from build123d import *

# Parameters (mm, degrees)
SKETCH_1_W                 = 40
SKETCH_1_H                 = 22
EXTRUDE_1_DEPTH            = 6
M3_TAPPED_HOLE1_AT_2_COUNT = 2
M3_TAPPED_HOLE1_AT_2_PITCH = 33
CHAMFER_1_SIZE             = 0.5
SKETCH_5_R                 = 7.5
CUT_EXTRUDE_2_DEPTH        = 12
CHAMFER1_SIZE              = 0.5
SKETCH2_W                  = 25
SKETCH2_H                  = 22
EXTRUDE2_DEPTH             = 6.5
CHAMFER2_SIZE              = 1
CHAMFER3_SIZE              = 3


with BuildPart() as part:
    # 草图1 → 拉伸1 (new, symmetric)
    with BuildSketch(Plane.XY):
        Rectangle(SKETCH_1_W, SKETCH_1_H)
    extrude(amount=EXTRUDE_1_DEPTH, both=True)

    # 草图4 → M3 Tapped Hole1 (revolve, cut)
    with BuildSketch(Plane(origin=(-16.5, -11, 3.5), x_dir=(0, 0, -1), z_dir=(1, 0, 0))):
        Polygon((0, 0), (0, 10.251075774), (1.25, 9.5), (1.25, 0), align=None)
    m3_tapped_hole1 = revolve(axis=Axis((-16.5, -17.35, 3.5), (0, 1, 0)), mode=Mode.SUBTRACT)

    # M3 Tapped Hole1 at 2: M3 Tapped Hole1 ×2
    with Locations(*[(i * M3_TAPPED_HOLE1_AT_2_PITCH, 0, 0) for i in range(1, M3_TAPPED_HOLE1_AT_2_COUNT)]):
        add(m3_tapped_hole1, mode=Mode.SUBTRACT)

    # 倒角1
    chamfer_1_edges = [part.edges().sort_by_distance(p)[0] for p in [
        (16.5, -11, 4.75),
        (-16.5, -11, 4.75),
    ]]
    chamfer(chamfer_1_edges, length=CHAMFER_1_SIZE)

    # 草图5 → 拉伸2 (cut)
    with BuildSketch(Plane.XY.offset(6)):
        Circle(SKETCH_5_R)
    extrude(amount=-CUT_EXTRUDE_2_DEPTH, mode=Mode.SUBTRACT)

    # Mirror1: M3 Tapped Hole1 across plane
    add(m3_tapped_hole1.mirror(Plane.XY), mode=Mode.SUBTRACT)

    # Mirror1 copy 1 sketch → Mirror1 copy 1 (revolve, cut)
    with BuildSketch(Plane(origin=(16.5, -11, -3.5), x_dir=(0, 0, 1), z_dir=(1, 0, 0))):
        Polygon((0, 0), (0, -10.251075774), (1.25, -9.5), (1.25, 0), align=None)
    revolve(axis=Axis((16.5, -17.35, -3.5), (0, -1, 0)), mode=Mode.SUBTRACT)

    # Chamfer1
    chamfer1_edges = [part.edges().sort_by_distance(p)[0] for p in [
        (16.5, -11, -4.75),
        (-16.5, -11, -4.75),
    ]]
    chamfer(chamfer1_edges, length=CHAMFER1_SIZE)

    # Sketch2 → Extrude2 (cut)
    with BuildSketch(Plane(origin=(0, 0, -6), x_dir=(-1, 0, 0), z_dir=(0, 0, -1))):
        Rectangle(SKETCH2_W, SKETCH2_H)
    extrude(amount=-EXTRUDE2_DEPTH, mode=Mode.SUBTRACT)

    # Chamfer2
    chamfer2_edges = [part.edges().sort_by_distance(p)[0] for p in [
        (12.5, 0, -6),
        (-12.5, 0, -6),
    ]]
    chamfer(chamfer2_edges, length=CHAMFER2_SIZE)

    # Chamfer3
    chamfer3_edges = [part.edges().sort_by_distance(p)[0] for p in [
        (20, 0, 6),
        (-20, 0, 6),
        (20, 0, -6),
        (-20, 0, -6),
    ]]
    chamfer(chamfer3_edges, length=CHAMFER3_SIZE)


solid = part.part
Geometry check sheet. Reference: the model listing, model coordinates, mm. A direction names the side the tool comes from. Give positions to 0.01 mm unless a question says otherwise; leave off trailing zeros. Order: outer loops, then holes, each group sorted by start corner. A loop starts at its lowest first (then second) coordinate and runs counter-clockwise, first axis right, second up.
1) Cross-section at C-C (z = -0.25). Record the boundary of the cut face in (x, y), then the cut area to 3 significant figures.
Results are:
outline: (-20, -11) - (-12.5, -11) - (-12.5, 11) - (-20, 11) - close; (12.5, -11) - (20, -11) - (20, 11) - (12.5, 11) - close
area: 330 mm2
2) Cross-section at A-A (x = 0). Record the boundary of the cut face in (y, z), then the cut area to 3 significant figures.
Results are:
outline: (-11, 0.5) - (-7.5, 0.5) - (-7.5, 6) - (-11, 6) - close; (7.5, 0.5) - (11, 0.5) - (11, 6) - (7.5, 6) - close
area: 38.5 mm2
3) Draft check along X on faces 4 (the conical face through (16.69, -0.88, 3.4)), 5 (the flat face through (-19, 0, 4)), 6 (the flat face through (-8, 0, 6)). Enter one of: released by +X, released by -X, zero draft, split by the parting line, or undercut.
Results are:
face 4: undercut
face 5: released by -X
face 6: zero draft
4) Gauge pin test, flat ends, axial feed: pin 1 (5 mm diameter, centred on x = -7.5, z = 0, fed in from +Y); pin 2 (9 mm diameter, centred on x = 0, y = 0, fed in from -Z); pin 3 (3 mm diameter, centred on x = 16.5, z = 3.5, fed in from -Y); pin 4 (11 mm diameter, centred on x = -1, y = 4.5, fed in from -Z). Record the tip position at first contact, or that the pin passes through.
Results are:
pin 1: stops at y = 11
pin 2: passes through
pin 3: stops at y = -10.75
pin 4: stops at z = 0.5
5) Tool access check on faces 1 (the flat face through (-13, -0.2, -5.5)), 2 (the flat face through (0, -11, 1)), 3 (the cylindrical face through (-17.554, -6.063, 2.828)). Record the directions out of +Z, -Z, +X, -X, +Y, -Y that give a thin tool (end or side, any length) a straight path to the whole face; none if there is none.
Results are:
face 1: -Z, +Y, -Y
face 2: +Z, -Z, +X, -X, -Y
face 3: -Y
6) Material ranges on probe 1 along Z at (x, y) = (-16.5, -6.75); probe 2 along X at (y, z) = (-5, 3.5); probe 3 along X at (y, z) = (-4, -3.5), recorded low to high.
Results are:
probe 1: z = -6 to -4.75, -2.25 to 2.25, 4.75 to 6
probe 2: x = -19.5 to -17.75, -15.25 to -5.59, 5.59 to 15.25, 17.75 to 19.5
probe 3: x = -19.5 to -17.75, -15.25 to -12.5, 12.5 to 15.25, 17.75 to 19.5
7) Cross-section at B-B (y = 0). Record the boundary of the cut face in (x, z), then the cut area to 3 significant figures.
Results are:
outline: (-20, -3) - (-17, -6) - (-13.5, -6) - (-12.5, -5) - (-12.5, 0.5) - (-7.5, 0.5) - (-7.5, 6) - (-17, 6) - (-20, 3) - close; (7.5, 0.5) - (12.5, 0.5) - (12.5, -5) - (13.5, -6) - (17, -6) - (20, -3) - (20, 3) - (17, 6) - (7.5, 6) - close
area: 216 mm2
8) Cross-section at D-D (y = -2.75). Record the boundary of the cut face in (x, z), then the cut area to 3 significant figures.
Results are:
outline: (-20, -3) - (-17, -6) - (-13.5, -6) - (-12.5, -5) - (-12.5, 0.5) - (-6.98, 0.5) - (-6.98, 6) - (-17, 6) - (-20, 3) - close; (6.98, 0.5) - (12.5, 0.5) - (12.5, -5) - (13.5, -6) - (17, -6) - (20, -3) - (20, 3) - (17, 6) - (6.98, 6) - close; hole circle Ø2.5 at (-16.5, -3.5); hole circle Ø2.5 at (-16.5, 3.5); hole circle Ø2.5 at (16.5, -3.5); hole circle Ø2.5 at (16.5, 3.5)
area: 202 mm2
